Autodesk Inventor part; units mm, degrees
ref_plane "Work Plane3" through (-5.6218, 26, -0.8451) normal (0, 0, -1) x (-1, 0, 0)
ref_plane "Work Plane2" through (7.7, 26, 0) normal (0, 0, 1) x (1, 0, 0)
ref_plane "Work Plane1" through (7.7, 26, 0) normal (0, 0, 1) x (1, 0, 0)
sketch "Sketch3" plane through (0, 0, 0) normal (0, 1, 0) x (-1, 0, 0)
  circle A0 centre (0, 0) radius 4.5
  circle A1 centre (0, 0) radius 2.6
  dimension "d10" = 9
  dimension "d11" = 5.2
extrude "Extrusion2" add sketch "Sketch3" along normal blind 4
sketch "Sketch4" plane through (0, 4, 0) normal (0, 1, 0) x (1, 0, 0)
  circle A0 centre (0, 0) radius 2.6
  line L0 (0, -2.6) -> (0, -1.6)
  line L1 (0, -1.6) -> (0, 2.6)
  line L2 (0, -1.6) -> (-2.0494, -1.6)
  line L3 (0, -1.6) -> (2.0494, -1.6)
  line L4 (0, 2.6) -> (0, 2.6)
  line L5 (0, 2.6) -> (0, 2.6)
  circle A1 centre (0, 0) radius 4.5
  circle A2 centre (0, 0) radius 2.6
  line L6 (0, 2.6) -> (0, 1.6)
  line L7 (0, 1.6) -> (2.0494, 1.6)
  line L8 (0, 1.6) -> (-2.0494, 1.6)
  point P0 (2.0494, 1.6)
  point P1 (-2.0494, 1.6)
  dimension "d14" = 1
  dimension "d20" = 1
extrude "Extrusion3" add sketch "Sketch4" along normal blind 6 contours L7 L1 A0 | A0 L0 L3 | L1 L8 A0 | A0 L2 L0 | A1
sketch "Sketch5" plane through (0, 10, 0) normal (0, 1, 0) x (1, 0, 0)
  circle A0 centre (0, 0) radius 4.5
extrude "Extrusion4" add sketch "Sketch5" along normal blind 1
sketch "Sketch11" plane through (0, 0, 0) normal (0, -1, 0) x (1, 0, 0)
  point P0 (0, 0)
sketch "Sketch12" plane through (0, 11, 0) normal (0, 1, 0) x (1, 0, 0)
  circle A0 centre (0, 0) radius 4.675
  circle A1 centre (0, 0) radius 5.685
  dimension "d59" = 9.35
  dimension "d60" = 11.37
extrude "Extrusion11" add sketch "Sketch12" along normal blind 2 contours A0 | A1
extrude "Extrusion12" add sketch "Sketch12" along normal blind 8
sketch "Sketch14" plane through (0, 19, 0) normal (0, 1, 0) x (1, 0, 0)
  point P0 (0, 0)
sketch "Sketch15" plane through (0, 19, 0) normal (0, 1, 0) x (1, 0, 0)
  circle A0 centre (0, 0) radius 5.685
  line L0 (5.685, 0) -> (5.585, 0)
  line L1 (5.585, 0) -> (5.585, -1.0616)
  circle A1 centre (0, 0) radius 5.685
  line L2 (5.585, 0) -> (5.585, 1.0616)
  line L3 (5.585, 1.0616) -> (12.585, 1.0616)
  line L4 (12.585, 1.0616) -> (12.585, -1.3379)
  line L5 (12.585, -1.3379) -> (5.585, -1.3379)
  line L6 (5.585, -1.3379) -> (5.585, 1.0616)
  line L7 (-5.6218, 0.8451) -> (-5.6218, -0.8451)
  line L8 (-5.6218, 0.8451) -> (-12.6218, 0.8451)
  line L9 (-12.6218, 0.8451) -> (-12.6218, -0.8451)
  line L10 (-12.6218, -0.8451) -> (-5.6218, -0.8451)
  line L11 (-5.6218, -0.8451) -> (-5.6218, 0.8451)
  point P0 (-5.6218, -0.8451)
  point P1 (8.9, -1.3379)
  point P2 (5.585, -1.0616)
  dimension "d72" = 0.1
  dimension "d73" = 7
  dimension "d74" = 7
ref_plane "Work Plane3" through (-5.6218, 26, -0.8451) normal (0, 0, -1) x (-1, 0, 0)
sketch "Sketch17" plane through (-5.6218, 26, -0.8451) normal (0, 0, -1) x (-1, 0, 0)
  line L0 (7, 0) -> (7, -7)
  line L1 (-10.3068, 0) -> (7, 0)
  line L2 (7, -3.5) -> (3.5, -3.5)
  line L3 (-18.2068, 0) -> (-18.2068, -7)
  line L4 (-18.2068, -3.5) -> (-14.7068, -3.5)
  point P0 (-5.6218, -26)
  dimension "d81" = 3.5
  dimension "d82" = 3.5
ref_plane "Work Plane2" through (7.7, 26, 0) normal (0, 0, 1) x (1, 0, 0)
sketch "Sketch19" plane through (7.7, 26, 0) normal (0, 0, 1) x (1, 0, 0)
  line L0 (-12.2, -26) -> (-12.2, -15)
  line L1 (-12.2, -26) -> (-19.2, -26)
  line L2 (-19.2, -26) -> (-19.2, -19)
  line L3 (-19.2, -19) -> (-12.2, -19)
  line L4 (-12.2, -19) -> (-12.2, -26)
  line L5 (-3.2, -15) -> (-3.2, -26)
  line L6 (-3.2, -26) -> (3.8, -26)
  line L7 (3.8, -26) -> (3.8, -19)
  line L8 (3.8, -19) -> (-3.2, -19)
  line L9 (-3.2, -19) -> (-3.2, -26)
  circle A0 centre (0.3, -22.5) radius 1.9558
  circle A1 centre (-15.7, -22.5) radius 1.9558
  point P0 (-7.7, -26)
  point P1 (-3.2, -19)
  dimension "d93" = 7
  dimension "d94" = 7
  dimension "d95" = 7
  dimension "d96" = 7
  dimension "d97" = 3.9116
  dimension "d98" = 3.9116
extrude "Extrusion17" add sketch "Sketch19" against normal blind 2
ref_plane "Work Plane1" through (7.7, 26, 0) normal (0, 0, 1) x (1, 0, 0)
sketch "Sketch20" plane through (7.7, 26, 0) normal (0, 0, 1) x (1, 0, 0)
  line L0 (-12.2, -19) -> (-12.2, -15)
  line L1 (-10.3, -16) -> (-10.3, -26)
  line L2 (-12.2, -19) -> (-10.3, -19)
  line L3 (-10.3, -19) -> (-10.3, -26)
  line L4 (-10.3, -26) -> (-12.2, -26)
  line L5 (-12.2, -26) -> (-12.2, -19)
  line L6 (-3.2, -26) -> (-5.1, -26)
  line L7 (-3.1953, -19) -> (-5.1, -19)
  line L8 (-5.1, -19) -> (-5.1, -26)
  line L9 (-5.1, -26) -> (-3.1953, -26)
  line L10 (-3.1953, -26) -> (-3.1953, -19)
  point P0 (-7.7, -26)
extrude "Extrusion18" add sketch "Sketch20" against normal blind 2
extrude "Extrusion20" add sketch "Sketch15" against normal blind 7 contours A0 L3 L4 L5 L6 | A0 L10 L9 L8
hole "Hole2" at (9.085, 22.5, -0.8451) at (-9.1218, 22.5, -0.8451) direction (0, 0, 1) diameter 3.4 end through all
sketch "Sketch22" plane through (7.7, 26, 0) normal (0, 0, 1) x (1, 0, 0)
  point P0 (-7.7, -26)
sketch "Sketch23" plane through (5.585, 19, 1.3379) normal (0, 0, 1) x (1, 0, 0)
  point P0 (-5.585, -19)
sketch "Sketch24" plane through (12.585, 19, -1.0616) normal (0, 0, -1) x (-1, 0, 0)
  line L0 (0, 0) -> (0, -7)
  line L1 (0, 0) -> (7, 0)
  line L2 (0, -3.5) -> (3.5, -3.5)
  line L3 (3.5, -3.5) -> (3.5, 0)
  line L4 (3.5, 0) -> (0, 0)
  line L5 (0, 0) -> (0, -3.5)
  line L6 (18.2068, 0) -> (25.2068, 0)
  line L7 (25.2068, 0) -> (21.7068, 0)
  line L8 (21.7068, 0) -> (21.7068, -3.5)
  line L9 (21.7068, -3.5) -> (25.2068, -3.5)
  line L10 (25.2068, -3.5) -> (25.2068, 0)
  point P0 (12.585, -19)
hole "Hole3" at (9.085, 15.5, -1.0616) at (-9.1218, 15.5, -1.0616) direction (0, 0, 1) diameter 3.4 end through all
sketch "Sketch21" plane through (0, 19, 0) normal (0, 1, 0) x (1, 0, 0)
  line L0 (12.585, 1.0616) -> (12.585, -1.3379)
  line L1 (12.585, -0.1382) -> (-17.8482, -0.1382)
  line L2 (-17.8482, -0.1382) -> (-17.8482, -11.8989)
  line L3 (-17.8482, -11.8989) -> (12.585, -11.8989)
  line L4 (12.585, -11.8989) -> (12.585, -0.1382)
  point P0 (0, 0)
extrude "Extrusion19" cut sketch "Sketch21" against normal blind 76.2
sketch "Sketch25" plane through (-12.6218, 19, 0.1382) normal (0, 0, 1) x (1, 0, 0)
  line L0 (7.9489, -6) -> (17.2948, -6)
  line L1 (17.2948, -6) -> (17.2948, -7)
  line L2 (25.2068, 0) -> (25.2068, -7)
  line L3 (17.2948, -7) -> (25.2068, -7)
  line L4 (25.2068, -7) -> (25.2068, 0)
  line L5 (25.2068, 0) -> (17.2948, 0)
  line L6 (17.2948, 0) -> (17.2948, -7)
  line L7 (7, 0) -> (0, 0)
  line L8 (7.9389, -7) -> (0, -7)
  line L9 (0, -7) -> (0, 0)
  line L10 (0, 0) -> (7.9389, 0)
  line L11 (7.9389, 0) -> (7.9389, -7)
  circle A0 centre (3.5, -3.5) radius 1.7
  circle A1 centre (21.7068, -3.5) radius 1.7
  point P0 (12.6218, -19)
extrude "Extrusion21" add sketch "Sketch25" against normal blind 2
sketch "Sketch26" plane through (7.7, 26, 0) normal (0, 0, 1) x (1, 0, 0)
  line L0 (-19.2, -26) -> (-12.2, -26)
  line L1 (-3.2, -26) -> (-3.2, -19)
  line L2 (-12.2, -19) -> (-19.2, -19)
  line L3 (-19.2, -19) -> (-19.2, -26)
  circle A0 centre (-15.7, -22.5) radius 1.9558
  circle A1 centre (0.3, -22.5) radius 1.9558
  line L4 (3.8, -26) -> (3.8, -19)
  line L5 (3.8, -19) -> (-3.2, -19)
  line L6 (-3.2, -26) -> (-3.2, -19)
  line L7 (-19.2, -26) -> (-12.2, -26)
  line L8 (-12.2, -26) -> (-12.2, -19)
  line L9 (-12.2, -19) -> (-19.2, -19)
  line L10 (-19.2, -19) -> (-19.2, -26)
  line L11 (-3.2, -26) -> (3.8, -26)
  line L12 (-12.2, -26) -> (-12.2, -19)
  line L13 (-3.2, -26) -> (3.8, -26)
  line L14 (3.8, -26) -> (3.8, -19)
  line L15 (3.8, -19) -> (-3.2, -19)
  point P0 (-7.7, -26)
extrude "Extrusion22" add sketch "Sketch26" along normal up to surface (0.1382 mm away)
properties part number "4"
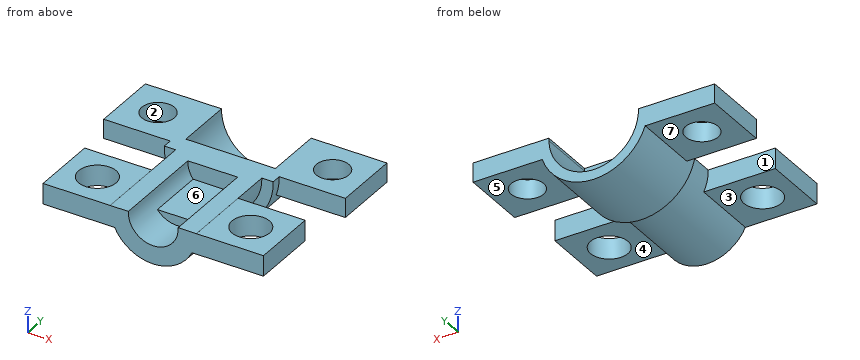
Design review of the part built by this model. Coordinates are the model's own, in mm. Face numbers are marked on the shaded views. A direction names the side the tool comes from. Round coordinates to 2 decimals unless told otherwise and drop trailing zeros. Order: outer loops, then holes, each group sorted by start corner. A loop starts at its lowest first (then second) coordinate and runs counter-clockwise, first axis right, second up.
1) Consider section C-C (x = -10.5). State the section outline as (y, z) points.
The answers:
outline: (0, -2) - (7, -2) - (7, 0.14) - (0, 0.14) - close; (12, -1.86) - (14.5, -1.86) - (14.5, 0.14) - (12, 0.14) - close; (16.5, -1.86) - (19, -1.86) - (19, 0.14) - (16.5, 0.14) - close
2) Clearance check with flat-ended pins moving along their axes: pin 1 Ø1.1 at (y, z) = (2.5, -0.5) entering from +X; pin 2 Ø2 at (x, y) = (9.5, 3) entering from -Z; pin 3 Ø1.2 at (x, y) = (0.5, 7.5) entering from +Z; pin 4 Ø1.5 at (x, z) = (9.5, -3.5) entering from +Y. State where each tip first meets the part, or that it passes through.
The answers:
pin 1: stops at x = 11.5
pin 2: stops at z = -2
pin 3: stops at z = -1.6
pin 4: passes through
3) Consider section D-D (z = -0.4). State the section outline as (x, y) points (3 decimals), plus the area to 3 significant figures.
The answers:
outline: (-12.622, 12) - (-5.671, 12) - (-5.671, 11) - (-4.482, 11) - (-4.482, 7) - (-11.5, 7) - (-11.5, 0) - (-2.569, 0) - (-2.569, 10) - (2.569, 10) - (2.569, 0) - (11.5, 0) - (11.5, 7) - (4.482, 7) - (4.482, 11) - (5.671, 11) - (5.671, 12) - (12.585, 12) - (12.585, 19) - (4.658, 19) - (4.658, 13) - (-4.658, 13) - (-4.658, 19) - (-12.622, 19) - close; hole circle Ø3.4 at (-9.122, 15.5); hole circle Ø3.912 at (-8, 3.5); hole circle Ø3.912 at (8, 3.5); hole circle Ø3.4 at (9.085, 15.5)
area: 235 mm2
4) Draft analysis for pull direction X (two halves, no side actions). For the marked faces 1 and 2, state which applies: released by +X, released by -X, zero draft, split by the parting line, or undercut.
The answers:
face 1: zero draft
face 2: undercut
5) Consider section B-B (y = 14.25). Count the separate pieces of the cut face and the enclosed holes in it, plus the area to 3 significant figures.
The answers:
separate pieces: 3
enclosed holes: 0
area: 35.6 mm2
6) For L1, parallel to Y at x = -6.5, z = -0.6; L2, parallel to X at y = 15.5, z = -0.65 (3 decimals); L3, parallel to Y at x = 8, z = -0.6, list the stretches that pass through material, from the lowest coordinate up.
The answers:
L1: y = 0 to 2.24, 4.76 to 7, 12 to 19
L2: x = -12.622 to -10.822, -7.422 to -4.63, 4.63 to 7.385, 10.785 to 12.585
L3: y = 0 to 1.54, 5.46 to 7, 12 to 14.19, 16.81 to 19
7) Machinability: for the marked faces 3, 4, 5, 6 and 7, which of the approach directions +Z, -Z, +X, -X, +Y, -Y give a long, thin tool a straight path to every point of the face, cutting with its end or side? Answer none if there is none.
The answers:
face 3: -Z, -X, -Y
face 4: -Z, +X, -Y
face 5: -Z, +X, +Y
face 6: +Z, -Y
face 7: -Z, -X, +Y
8) Consider section A-A (x = 8). State the section outline as (y, z) points.
The answers:
outline: (0, -2) - (1.54, -2) - (1.54, 0.14) - (0, 0.14) - close; (5.46, -2) - (7, -2) - (7, 0.14) - (5.46, 0.14) - close; (12, -1.86) - (14.19, -1.86) - (14.19, 0.14) - (12, 0.14) - close; (16.81, -1.86) - (19, -1.86) - (19, 0.14) - (16.81, 0.14) - close
